from build123d import *

# Parameters (mm, degrees)
F0_W      = 55
F0_H      = 50
F0_R      = 3.5
F0_R_2    = 1.725
F1_DEPTH  = 4
F2_R      = 3.5
F3_DEPTH  = 2
F5_DEPTH  = 22
F6_R      = 5.25
F6_R_2    = 1.725
F7_DEPTH  = 6
F8_W      = 55
F8_H      = 50
F9_DEPTH  = 4
F10_R     = 2
F11_R     = 1.725
F12_DEPTH = 4
F14_DEPTH = 2
F15_R     = 3
F16_DEPTH = 4.2689492924


with BuildPart() as f1:
    # F0 (on Top) → F1 (new body)
    with BuildSketch(Plane.XY):
        with Locations((27.5, 25)):
            Rectangle(F0_W, F0_H)
        with Locations((17.5, 15)):
            Circle(F0_R, mode=Mode.SUBTRACT)
        with Locations((37.5, 15)):
            Circle(F0_R, mode=Mode.SUBTRACT)
        with Locations((17.5, 35)):
            Circle(F0_R, mode=Mode.SUBTRACT)
        with Locations((37.5, 35)):
            Circle(F0_R, mode=Mode.SUBTRACT)
        with Locations((17.5, 35)):
            Circle(F0_R)
        with Locations((17.5, 35)):
            Circle(F0_R_2, mode=Mode.SUBTRACT)
        with Locations((37.5, 35)):
            Circle(F0_R)
        with Locations((37.5, 35)):
            Circle(F0_R_2, mode=Mode.SUBTRACT)
        with Locations((37.5, 15)):
            Circle(F0_R)
        with Locations((37.5, 15)):
            Circle(F0_R_2, mode=Mode.SUBTRACT)
        with Locations((17.5, 15)):
            Circle(F0_R)
        with Locations((17.5, 15)):
            Circle(F0_R_2, mode=Mode.SUBTRACT)
    extrude(amount=F1_DEPTH)

    # F2 (on face) → F3 (cut)
    with BuildSketch(Plane.XY.offset(4)):
        with Locations((17.5, 35)):
            Circle(F2_R)
        with Locations((37.5, 35)):
            Circle(F2_R)
        with Locations((37.5, 15)):
            Circle(F2_R)
        with Locations((17.5, 15)):
            Circle(F2_R)
    extrude(amount=-F3_DEPTH, mode=Mode.SUBTRACT)

    # F4 (on face) → F5 (join)
    with BuildSketch(Plane.XY.offset(4)):
        Polygon((4, 50), (0, 50), (0, 0), (55, 0), (55, 50), (51, 50), (51, 6), (4, 6), align=None)
    extrude(amount=F5_DEPTH)

    # F6 (on face) → F7 (cut, through all)
    with BuildSketch(Plane(origin=(0, 6, 0), x_dir=(-1, 0, 0), z_dir=(0, 1, 0))):
        with Locations((-40, 15)):
            Circle(F6_R)
        with Locations((-15, 22.6)):
            Circle(F6_R_2)
        with Locations((-15, 7.4)):
            Circle(F6_R_2)
        with Locations((-15, 15)):
            Circle(F6_R)
    extrude(amount=-F7_DEPTH, mode=Mode.SUBTRACT)

    # F8 (on face) → F9 (join)
    with BuildSketch(Plane.XY.offset(26)):
        with Locations((27.5, 25)):
            Rectangle(F8_W, F8_H)
    extrude(amount=F9_DEPTH)

    # F10
    f10_edges = [f1.edges().sort_by_distance(p)[0] for p in [
        (0, 25, 30),
        (0, 25, 0),
        (55, 25, 0),
        (55, 25, 30),
        (51, 28, 26),
        (4, 28, 26),
        (4, 28, 4),
        (51, 28, 4),
    ]]
    fillet(f10_edges, radius=F10_R)

    # F11 (on face) → F12 (cut, through all)
    with BuildSketch(Plane.XY.offset(30)):
        with Locations((17.5, 35)):
            Circle(F11_R)
        with Locations((37.5, 35)):
            Circle(F11_R)
        with Locations((37.5, 15)):
            Circle(F11_R)
        with Locations((17.5, 15)):
            Circle(F11_R)
    extrude(amount=-F12_DEPTH, mode=Mode.SUBTRACT)

    # F13 (on face) → F14 (cut)
    with BuildSketch(Plane(origin=(0, 0, 26), x_dir=(1, 0, 0), z_dir=(0, 0, -1))):
        Polygon((20.26, -13.406513257), (17.5, -11.8130265141), (14.74, -13.406513257), (14.74, -16.593486743), (17.5, -18.1869734859), (20.26, -16.593486743), align=None)
        Polygon((40.26, -13.406513257), (37.5, -11.8130265141), (34.74, -13.406513257), (34.74, -16.593486743), (37.5, -18.1869734859), (40.26, -16.593486743), align=None)
        Polygon((40.26, -33.406513257), (37.5, -31.8130265141), (34.74, -33.406513257), (34.74, -36.593486743), (37.5, -38.1869734859), (40.26, -36.593486743), align=None)
        Polygon((20.26, -33.406513257), (17.5, -31.8130265141), (14.74, -33.406513257), (14.74, -36.593486743), (17.5, -38.1869734859), (20.26, -36.593486743), align=None)
    extrude(amount=-F14_DEPTH, mode=Mode.SUBTRACT)

    # F15 (on face) → F16 (cut, through all)
    with BuildSketch(Plane.XY.offset(30)):
        with Locations((8, 25)):
            Circle(F15_R)
        with Locations((47, 25)):
            Circle(F15_R)
    extrude(amount=-F16_DEPTH, mode=Mode.SUBTRACT)


solid = f1.part
Model file for the job. Use its own axes, mm. A direction names the side the tool comes from. Give positions to 0.01 mm unless a question says otherwise; leave off trailing zeros. Order: outer loops, then holes, each group sorted by start corner. A loop starts at its lowest first (then second) coordinate and runs counter-clockwise, first axis right, second up. Notation, with made-up numbers: M 6,57.25 L 19,57.25 A13 cw 19,80.25 Z; hole C 19.5,20.5 d5. An arc over 180 degrees is marked long. Put each result on its own line as item: value. Start each with the question number.
(1) Band-saw the part on A-A on z = 7.4. Give the cut face in (x, y) (3 decimals), then the cut area to 3 significant figures.
(2) Pin check, flat tips, straight feed: pin 1 Ø5.5 at (x, y) = (37.5, 35) entering from +Z; pin 2 Ø2 at (x, z) = (38.5, 9) entering from +Y. Stop position of each tip, or through.
(3) Band-saw the part on C-C on y = 39.5. Give the cut face in (x, z), then the cut area to 3 significant figures.
(4) Band-saw the part on B-B on x = 47. Give the cut face in (y, z).
(5) Drill centre lines: L1, parallel to Y at x = 17.5, z = 1.15 (3 decimals); L2, parallel to Y at x = 47, z = 27.2; L3, parallel to Z at x = 45, y = 7.5. Where is each one in solid material? Low to high. Write a range as [from, to].
(6) Tool access for faces 1 (the face through (37.126, 33.316, 29.014)), 2 (the face through (40.26, 15, 27)), 3 (the face through (5, 25, 28)), 4 (the face through (4.57, 28.31, 25.4)): list every direction of +Z, -Z, +X, -X, +Y, -Y with a clear straight run to the whole face (end or side of a thin tool).
(7) Pull direction Z, two halves, no side cores. Call faces 5 (the face through (36.14, 32.6, 26.99)), 6 (the face through (27, 25, 30)), 7 (the face through (55, 25, 15)): released by +Z, released by -Z, zero draft, split by the parting line, or undercut.
(8) Band-saw the part on D-D on y = 15. Count the separate pieces of the cut face and the enclosed holes in it, then the cut area to 3 significant figures.
Results below:
1. outline: M 0,0 L 13.275,0 L 13.275,6 L 4,6 L 4,50 L 0,50 Z; M 16.725,0 L 55,0 L 55,50 L 51,50 L 51,6 L 16.725,6 Z
1. area: 661 mm2
2. pin 1: stops at z = 30
2. pin 2: stops at y = 6
3. outline: M 0,2 A2 ccw 2,0 L 53,0 A2 ccw 55,2 L 55,28 A2 ccw 53,30 L 2,30 A2 ccw 0,28 Z; hole M 4,6 A2 ccw 6,4 L 49,4 A2 ccw 51,6 L 51,24 A2 ccw 49,26 L 6,26 A2 ccw 4,24 Z
3. area: 616 mm2
4. outline: M 0,0 L 50,0 L 50,4 L 6,4 L 6,26 L 22,26 L 22,30 L 0,30 Z; M 28,26 L 50,26 L 50,30 L 28,30 Z
5. L1: y = [0, 13.275], [16.725, 33.275], [36.725, 50]
5. L2: y = [0, 22], [28, 50]
5. L3: z = [0, 4], [26, 30]
6. face 1: +Z, -Z
6. face 2: none
6. face 3: +Z
6. face 4: +Y
7. face 5: undercut
7. face 6: released by +Z
7. face 7: zero draft
8. separate pieces: 4
8. enclosed holes: 0
8. area: 538 mm2
